Model file for the job. Use its own axes, mm. Face numbers are marked on the shaded views. Round coordinates to 2 decimals unless told otherwise and drop trailing zeros. Loops run counter-clockwise (first coordinate to the right, second up) from the corner with the lowest first, then second, coordinate; pieces in that order, holes last. Notation, with made-up numbers: M -10,52 L 41,52 A24 cw 41,86 Z; hole C 12,-2.75 d10. An arc over 180 degrees is marked long. Use a Markdown table: item, result. Add a question column.
Q1. Probe line 1 (Y direction, x = 21, z = 10); line 2 (Z direction, x = 23.5, y = -60.5); line 3 (Y direction, x = 2, z = 18). List the from-to ranges inside material, lowest first. Write a range as from..to.
Q2. Mould opens along Z. For the marked faces 1, 2, 3 and 4 say: +Z half, -Z half, draft (parallel to the pull), parting line (faces both ways), or undercut.
Q3. Cut at A-A (z = 47.5). Give the cut face in (x, y) (3 decimals), plus the area to 3 significant figures.
Q4. Cut at D-D (z = 10). Give the cut face in (x, y).
Q5. Cut at C-C (y = -65.5). Give the cut face in (x, z).
Q6. Cut at B-B (x = 24.5). Give the cut face in (y, z).
Q7. Pin check, flat tip, straight feed: pin 1 (1 mm diameter, centred on x = 22, z = 44, fed in from +Y) (3 decimals). Stop position of the tip, or through.
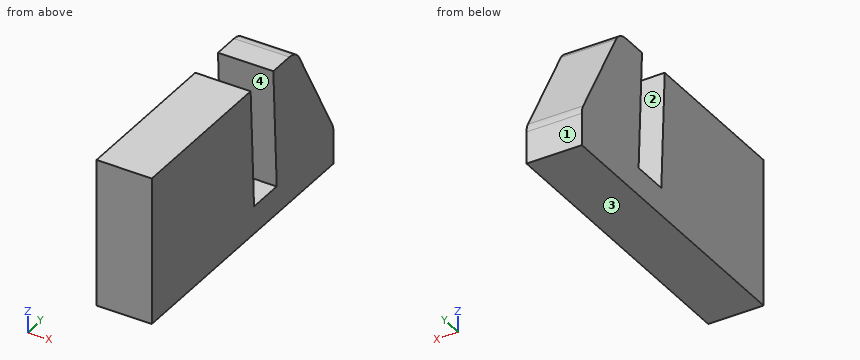
from build123d import *

# Parameters (mm, degrees)
F1_DEPTH = 30
F2_R     = 10


with BuildPart() as f1:
    # F0 (on Right) → F1 (new body)
    with BuildSketch(Plane.YZ):
        Polygon((-160, 65), (-160, 0), (-160, -15), (0, -15), (0, 5), (-33, 65), (-53, 65), (-50, 0), (-70, 0), (-73, 65), align=None)
    extrude(amount=F1_DEPTH)

    # F2
    f2_edges = [f1.edges().sort_by_distance(p)[0] for p in [
        (15, -33, 65),
        (15, 0, 5),
    ]]
    fillet(f2_edges, radius=F2_R)


solid = f1.part
Checked values:
| question | item | result |
|---|---|---|
| 1 | line 1 | y = -160..-70.46, -50.46..-2.75 |
| 1 | line 2 | z = -15..0 |
| 1 | line 3 | y = -160..-70.83, -50.83..-7.15 |
| 2 | face 1 | draft |
| 2 | face 2 | +Z half |
| 2 | face 3 | -Z half |
| 2 | face 4 | undercut |
| 3 | outline | M 0,-160 L 30,-160 L 30,-72.192 L 0,-72.192 Z; M 0,-52.192 L 30,-52.192 L 30,-23.375 L 0,-23.375 Z |
| 3 | area | 3,500 mm^2 |
| 4 | outline | M 0,-160 L 30,-160 L 30,-70.46 L 0,-70.46 Z; M 0,-50.46 L 30,-50.46 L 30,-2.75 L 0,-2.75 Z |
| 5 | outline | M 0,-15 L 30,-15 L 30,0 L 0,0 Z |
| 6 | outline | M -160,-15 L 0,-15 L 0,2.43 A10 ccw -1.24,7.25 L -30.15,59.82 A10 ccw -38.91,65 L -53,65 L -50,0 L -70,0 L -73,65 L -160,65 Z |
| 7 | pin 1 | stops at y = -21.175 |
